from build123d import *

# Parameters (mm, degrees)
F0_W     = 101.286828
F0_H     = 68.889946
F1_DEPTH = 45.275418
F2_R     = 50.358539


with BuildPart() as f1:
    # F0 (on Right) → F1 (new body)
    with BuildSketch(Plane.YZ):
        with Locations((14.08571, 0)):
            Rectangle(F0_W, F0_H)
    extrude(amount=F1_DEPTH)

    # F2
    f2_edges = [f1.edges().sort_by_distance(p)[0] for p in [
        (22.637709, -36.557704, 34.444973),
    ]]
    fillet(f2_edges, radius=F2_R)


solid = f1.part
Work out the finished part from the listing and answer in its coordinate system (mm). Give positions to 0.01 mm unless a question says otherwise; leave off trailing zeros. Loops run counter-clockwise (first coordinate to the right, second up) from the corner with the lowest first, then second, coordinate; pieces in that order, holes last. Notation, with made-up numbers: (-19.75, -38.75) - (18.25, -38.75) arc R22 ccw to (18.25, -6.75) - close; hole circle Ø7 at (58.25, 27). An arc over 180 degrees is marked (long way). Answer in a Markdown table with one row per item. Add a question column.
Q1. The part is cut by section A-A (x = 41). Determine the outline of the cut face in (y, z), and give its area (3 significant figures).
Q2. The part is cut by section C-C (y = -18.5). Determine the outline of the cut face in (x, z), and give its area (3 significant figures).
Q3. Consider line 1 along Z through (x, y) = (28, 13); line 2 along Y through (x, z) = (5.5, 27); line 3 along Z through (x, y) = (10, -4). Determine where each line is inside the solid, lowest interval first.
Q4. The part is cut by section B-B (z = 17.5). Determine the outline of the cut face in (x, y).
Solution:
| question | item | result |
|---|---|---|
| 1 | outline | (-36.56, -34.44) - (64.73, -34.44) - (64.73, 34.44) - (13.8, 34.44) arc R50.36 ccw to (-36.56, -15.91) - close |
| 1 | area | 6,430 mm² |
| 2 | outline | (0, -34.44) - (45.28, -34.44) - (45.28, 22.72) - (0, 22.72) - close |
| 2 | area | 2,590 mm² |
| 3 | line 1 | z = -34.44 to 34.44 |
| 3 | line 2 | y = -12.55 to 64.73 |
| 3 | line 3 | z = -34.44 to 31.19 |
| 4 | outline | (0, -23.88) - (45.28, -23.88) - (45.28, 64.73) - (0, 64.73) - close |
